Build history of the part. All positions in model axes, mm. Face numbers are marked on the shaded views. Give positions to 0.01 mm unless a question says otherwise; leave off trailing zeros. Loops run counter-clockwise (first coordinate to the right, second up) from the corner with the lowest first, then second, coordinate; pieces in that order, holes last.
1) Band-saw the part on A-A on y = -50. List the corners of the cut face in (x, z).
2) Two-plate mould, pull along Y, no slides. Class the marked faces 1 and 2: +Y half, -Y half, draft (parallel to the pull), parting line (faces both ways), or undercut.
3) Wall check: line 1 (Y direction, x = 0, z = 10) (3 decimals); line 2 (X direction, y = 45.5, z = 4.25); line 3 (Y direction, x = 8, z = 1.75). Give the ranges that are in metal, low to high.
4) Flat gauge pin, fed straight in: P1, Ø15.5, axis at x = 0, y = 42.5, coming from the -Z side. Where does the tip first touch, or does it go through?
5) Band-saw the part on D-D on y = 42.5. List the corners of the cut face in (x, z) (3 decimals), then the cut area to 3 significant figures.
6) Band-saw the part on B-B on x = 0. List the corners of the cut face in (y, z) (3 decimals).
7) Band-saw the part on C-C on z = 11. List the corners of the cut face in (x, y) (3 decimals), then the cut area to 3 significant figures.
```python
from build123d import *

# Parameters (mm, degrees)
SKETCH2_W                  = 160
SKETCH2_H                  = 180
BOSS_EXTRUDE1_DEPTH        = 15
F_20_0_20_DIAMETER_HOLE1_D = 26.01
F_6_0MM_DOWEL_HOLE1_D      = 6
F_6_0MM_DOWEL_HOLE1_DEPTH  = 40
F_6_0MM_DOWEL_HOLE1_TIP    = 1.802581857
SKETCH10_R                 = 12.7
CUT_EXTRUDE1_DEPTH         = 16


with BuildPart() as part:
    # Sketch2 → Boss-Extrude1 (new body)
    with BuildSketch(Plane.XY):
        with Locations((0, -5)):
            Rectangle(SKETCH2_W, SKETCH2_H)
    extrude(amount=BOSS_EXTRUDE1_DEPTH)

    # Ø20.0 (20) Diameter Hole1 (through all)
    with Locations(Plane.XY.offset(15)):
        with Locations((0, 42.5)):
            Hole(F_20_0_20_DIAMETER_HOLE1_D / 2)

    # Ø6.0mm Dowel Hole1
    with Locations(Plane.XY.offset(15)):
        with Locations((0, 8.5)):
            Hole(F_6_0MM_DOWEL_HOLE1_D / 2, depth=F_6_0MM_DOWEL_HOLE1_DEPTH)
            with Locations((0, 0, -(F_6_0MM_DOWEL_HOLE1_DEPTH + F_6_0MM_DOWEL_HOLE1_TIP / 2))):  # 118° drill point
                Cone(0, F_6_0MM_DOWEL_HOLE1_D / 2, F_6_0MM_DOWEL_HOLE1_TIP, mode=Mode.SUBTRACT)

    # Sketch10 → Cut-Extrude1 (cut, through all)
    with BuildSketch(Plane.XY.offset(15)):
        with Locations((0, -50)):
            Circle(SKETCH10_R)
    extrude(amount=-CUT_EXTRUDE1_DEPTH, mode=Mode.SUBTRACT)


solid = part.part
```
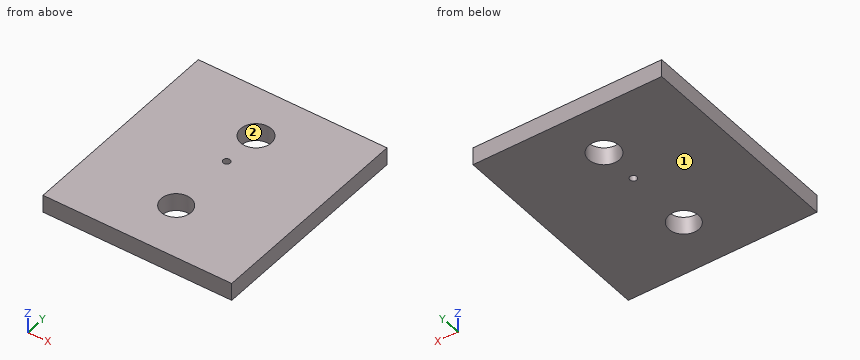
Findings below:
1. outline: (-80, 0) - (-12.7, 0) - (-12.7, 15) - (-80, 15) - close; (12.7, 0) - (80, 0) - (80, 15) - (12.7, 15) - close
2. face 1: draft
2. face 2: undercut
3. line 1: y = -95 to -62.7, -37.3 to 5.5, 11.5 to 29.495, 55.505 to 85
3. line 2: x = -80 to -12.65, 12.65 to 80
3. line 3: y = -95 to -59.86, -40.14 to 32.25, 52.75 to 85
4. P1: passes through
5. outline: (-80, 0) - (-13.005, 0) - (-13.005, 15) - (-80, 15) - close; (13.005, 0) - (80, 0) - (80, 15) - (13.005, 15) - close
5. area: 2,010 mm2
6. outline: (-95, 0) - (-62.7, 0) - (-62.7, 15) - (-95, 15) - close; (-37.3, 0) - (5.5, 0) - (5.5, 15) - (-37.3, 15) - close; (11.5, 0) - (29.495, 0) - (29.495, 15) - (11.5, 15) - close; (55.505, 0) - (85, 0) - (85, 15) - (55.505, 15) - close
7. outline: (-80, -95) - (80, -95) - (80, 85) - (-80, 85) - close; hole circle Ø26.01 at (0, 42.5); hole circle Ø25.4 at (0, -50); hole circle Ø6 at (0, 8.5)
7. area: 27,700 mm2
